For this review, take the finished solid that the model builds, in its own axes (mm). A direction names the side the tool comes from. Round coordinates to 2 decimals unless told otherwise and drop trailing zeros. Order: outer loops, then holes, each group sorted by start corner. A loop starts at its lowest first (then second) coordinate and runs counter-clockwise, first axis right, second up. Notation, with made-up numbers: (64.25, -6.5) -> (100.25, -6.5) arc R11 ccw to (100.25, 9.5) -> close; hole circle Ø6 at (70.25, 85). An arc over 180 degrees is marked (long way). Answer in a Markdown table with one row per item.
```python
from build123d import *

# Parameters (mm, degrees)
SKETCH1_W                = 18
SKETCH1_H                = 21
BOSS_EXTRUDE1_DEPTH      = 20
CUT_EXTRUDE3_DEPTH       = 30
CUT_EXTRUDE4_DEPTH       = 27
SKETCH6_W                = 20
SKETCH6_H                = 17
CUT_EXTRUDE5_DEPTH       = 17
SKETCH9_W                = 17
SKETCH9_H                = 4
CUT_EXTRUDE7_DEPTH       = 4
SKETCH10_W               = 20
SKETCH10_H               = 4
CUT_EXTRUDE8_DEPTH       = 30
BOSS_EXTRUDE3_DEPTH      = 4
SKETCH13_W               = 18
SKETCH13_H               = 1.5
SKETCH13_W_2             = 20
CUT_EXTRUDE11_DEPTH      = 21
CUT_EXTRUDE12_DEPTH      = 26
SKETCH16_R               = 1.9
BOSS_EXTRUDE4_DEPTH      = 14.5
SKETCH22_R               = 1.25
CUT_EXTRUDE15_DEPTH      = 19
CUT_EXTRUDE15_DEPTH_BACK = 27
CHAMFER1_SIZE            = 1.5
SKETCH23_W               = 18
SKETCH23_H               = 5
CUT_EXTRUDE16_DEPTH      = 4
SKETCH24_R               = 2
BOSS_EXTRUDE7_DEPTH      = 29
BOSS_EXTRUDE8_REACH      = 31
SKETCH25_W               = 4.5
SKETCH25_H               = 5.9
SKETCH26_R               = 1.6
CUT_EXTRUDE17_DEPTH      = 10


with BuildPart() as part:
    # Sketch1 → Boss-Extrude1 (new body)
    with BuildSketch(Plane(origin=(0, 0, 0), x_dir=(1, 0, 0), z_dir=(0, 1, 0))):
        Polygon((17.5, 14.5), (-8.5, 14.5), (-8.5, -14.5), (17.5, -14.5), (17.5, -10.5), (17.5, 10.5), align=None)
        with Locations((26.5, 0)):
            Rectangle(SKETCH1_W, SKETCH1_H)
    extrude(amount=BOSS_EXTRUDE1_DEPTH)

    # Sketch3 → Cut-Extrude3 (cut, through all)
    with BuildSketch(Plane.XY.offset(14.5)):
        Polygon((-8.5, 20), (-8.5, 18.5), (-4.5, 20), align=None)
    extrude(amount=-CUT_EXTRUDE3_DEPTH, mode=Mode.SUBTRACT)

    # Sketch4 → Cut-Extrude4 (cut, through all)
    with BuildSketch(Plane(origin=(17.5, 0, 0), x_dir=(0, 0, -1), z_dir=(1, 0, 0))):
        Polygon((-14.5, 20), (-14.5, 18.5), (-11.5, 20), align=None)
        Polygon((14.5, 20), (11.5, 20), (14.5, 18.5), align=None)
    extrude(amount=-CUT_EXTRUDE4_DEPTH, mode=Mode.SUBTRACT)

    # Sketch6 → Cut-Extrude5 (cut)
    with BuildSketch(Plane.XZ):
        with Locations((4.5, 0)):
            Rectangle(SKETCH6_W, SKETCH6_H)
    extrude(amount=-CUT_EXTRUDE5_DEPTH, mode=Mode.SUBTRACT)

    # Sketch9 → Cut-Extrude7 (cut)
    with BuildSketch(Plane.ZY.offset(8.5)):
        with Locations((0, 15)):
            Rectangle(SKETCH9_W, SKETCH9_H)
    extrude(amount=-CUT_EXTRUDE7_DEPTH, mode=Mode.SUBTRACT)

    # Sketch10 → Cut-Extrude8 (cut, through all)
    with BuildSketch(Plane.XY.offset(14.5)):
        with Locations((4.5, 12)):
            Rectangle(SKETCH10_W, SKETCH10_H)
    extrude(amount=-CUT_EXTRUDE8_DEPTH, mode=Mode.SUBTRACT)

    # Sketch12 → Boss-Extrude3 (add)
    with BuildSketch(Plane.XY.offset(14.5)):
        Polygon((22.5, 1.4), (34.5, 1.4), (34.5, 0), (34.5, -2), (29.5, -5), (12.5, -5), (7.5, 0), (17.5, 0), (17.5, 5), align=None)
    boss_extrude3 = extrude(amount=-BOSS_EXTRUDE3_DEPTH)

    # Mirror1: Boss-Extrude3 across plane
    add(boss_extrude3.mirror(Plane.XY))

    # Sketch13 → Cut-Extrude11 (cut)
    with BuildSketch(Plane.XY.offset(10.5)):
        with Locations((26.5, 19.25)):
            Rectangle(SKETCH13_W, SKETCH13_H)
        with Locations((25.5, 0.75)):
            Rectangle(SKETCH13_W_2, SKETCH13_H)
    extrude(amount=-CUT_EXTRUDE11_DEPTH, mode=Mode.SUBTRACT)

    # Sketch14 → Cut-Extrude12 (cut, through all)
    with BuildSketch(Plane.XY.offset(10.5)):
        with BuildLine():
            ThreePointArc((35.5, 10), (33.01040764, 3.98959236), (27, 1.5))
            Line((27, 1.5), (35.5, 1.5))
            Line((35.5, 1.5), (35.5, 10))
        make_face()
        with BuildLine():
            Line((35.5, 18.5), (27, 18.5))
            ThreePointArc((27, 18.5), (33.01040764, 16.01040764), (35.5, 10))
            Line((35.5, 10), (35.5, 18.5))
        make_face()
    extrude(amount=-CUT_EXTRUDE12_DEPTH, mode=Mode.SUBTRACT)

    # Sketch16 → Boss-Extrude4 (add, symmetric)
    with BuildSketch(Plane.XY):
        with Locations((27, 10)):
            Circle(SKETCH16_R)
    extrude(amount=BOSS_EXTRUDE4_DEPTH, both=True)

    # Sketch22 → Cut-Extrude15 (cut, two sides)
    with BuildSketch(Plane(origin=(17.5, 0, 0), x_dir=(0, 0, -1), z_dir=(1, 0, 0))) as cut_extrude15_sk:
        with Locations((0, 15.75)):
            Circle(SKETCH22_R)
    extrude(amount=CUT_EXTRUDE15_DEPTH, mode=Mode.SUBTRACT)
    extrude(cut_extrude15_sk.sketch, amount=-CUT_EXTRUDE15_DEPTH_BACK, mode=Mode.SUBTRACT)

    # Chamfer1
    chamfer1_edges = [part.edges().sort_by_distance(p)[0] for p in [
        (22.25, 18.5, -10.5),
        (22.25, 18.5, 10.5),
        (24.680555556, 1.5, 10.5),
        (24.680555556, 1.5, -10.5),
        (35.5, 10, -10.5),
        (35.5, 10, 10.5),
    ]]
    chamfer(chamfer1_edges, length=CHAMFER1_SIZE)

    # Sketch23 → Cut-Extrude16 (cut)
    with BuildSketch(Plane(origin=(0, 18.5, 0), x_dir=(1, 0, 0), z_dir=(0, 1, 0))):
        with Locations((26.5, 0)):
            Rectangle(SKETCH23_W, SKETCH23_H)
    extrude(amount=-CUT_EXTRUDE16_DEPTH, mode=Mode.SUBTRACT)

    # Sketch24 → Boss-Extrude7 (add, through all)
    with BuildSketch(Plane.XY.offset(14.5)):
        with Locations((3.5, 0)):
            Circle(SKETCH24_R)
    extrude(amount=-BOSS_EXTRUDE7_DEPTH)

    # Sketch25 → Boss-Extrude8 (add, up to next)
    with BuildSketch(Plane.XY.offset(14.5), mode=Mode.PRIVATE) as boss_extrude8_sk1:
        with Locations((27.25, -2.05)):
            Rectangle(SKETCH25_W, SKETCH25_H)
    boss_extrude8_tool1 = extrude(boss_extrude8_sk1.sketch, amount=-BOSS_EXTRUDE8_REACH, mode=Mode.PRIVATE) - part.part
    add(boss_extrude8_tool1.solids().sort_by_distance((27.25, -2.05, 14.5))[0])

    # Sketch26 → Cut-Extrude17 (cut)
    with BuildSketch(Plane(origin=(29.5, 0, 0), x_dir=(0, 0, -1), z_dir=(1, 0, 0))):
        with Locations((0, -2.05)):
            Circle(SKETCH26_R)
    extrude(amount=-CUT_EXTRUDE17_DEPTH, mode=Mode.SUBTRACT)


solid = part.part
```
Q1. Take a section at A-A, the plane x = 3.5. Write out the cut boundary in (y, z), then the cut area to 4 significant figures.
Answer key:
| item | result |
|---|---|
| outline | (-2, -14.5) -> (10, -14.5) -> (10, -8.5) -> (2, -8.5) -> (2, 8.5) -> (10, 8.5) -> (10, 14.5) -> (-2, 14.5) -> close; (14, -14.5) -> (18.5, -14.5) -> (20, -11.5) -> (20, 11.5) -> (18.5, 14.5) -> (14, 14.5) -> (14, 8.5) -> (17, 8.5) -> (17, -8.5) -> (14, -8.5) -> close |
| area | 330.5 mm^2 |
Q2. Tool access review of faces 1 (the face through (4, 10, -11)), 2 (the face through (21, 1.5, 0)), 3 (the face through (25, 0, 0)), 4 (the face through (26, 14.5, 0)), 5 (the face through (14.5, 8, 0)): name each direction out of +Z, -Z, +X, -X, +Y, -Y from which nothing blocks a thin tool from reaching the whole face with its end or side.
Answer key:
| item | result |
|---|---|
| face 1 | +Z, -Z |
| face 2 | +X |
| face 3 | -Y |
| face 4 | +X, +Y |
| face 5 | none |
Q3. Clearance check with flat-ended pins moving along their axes: pin 1 Ø13.5 at (x, z) = (1.5, 0) entering from -Y; pin 2 Ø3 at (x, y) = (26.5, 16) entering from +Z; pin 3 Ø1 at (y, z) = (0, 13) entering from +X. State where each tip first meets the part, or that it passes through.
Answer key:
| item | result |
|---|---|
| pin 1 | stops at y = -2 |
| pin 2 | stops at z = 10.5 |
| pin 3 | stops at x = 34.5 |
Q4. The part is to be moulded in two halves that separate along Y. For faces 6 (the face through (29.5, 0, 0)), 7 (the face through (22, 18.5, 6)), 8 (the face through (28, 1.4, 13)), say which applies: +Y half, -Y half, draft (parallel to the pull), parting line (faces both ways), or undercut.
Answer key:
| item | result |
|---|---|
| face 6 | draft |
| face 7 | +Y half |
| face 8 | undercut |
Q5. To check wall thickness, follow probe 1 along Y at (x, z) = (26.05, 0); probe 2 along Z at (x, y) = (13, 14.75); probe 3 along Z at (x, y) = (15.95, 15.75). State the ranges of each line that lie inside material, in increasing order.
Answer key:
| item | result |
|---|---|
| probe 1 | y = -5 to -3.65, -0.45 to 0.9, 1.5 to 14.5 |
| probe 2 | z = -14.5 to -8.5, 8.5 to 14.5 |
| probe 3 | z = -14.5 to -1.25, 1.25 to 14.5 |
Q6. Take a section at D-D, the plane x = 31. Give the number of separate pieces and of enclosed holes in the cut face, then the cut area to 3 significant figures.
Answer key:
| item | result |
|---|---|
| separate pieces | 3 |
| enclosed holes | 0 |
| area | 339 mm^2 |
Q7. Take a section at C-C, the plane x = 16. Write out the cut boundary in (y, z).
Answer key:
| item | result |
|---|---|
| outline | (-5, -14.5) -> (18.5, -14.5) -> (20, -11.5) -> (20, 11.5) -> (18.5, 14.5) -> (-5, 14.5) -> (-5, 10.5) -> (1.5, 10.5) -> (1.5, -10.5) -> (-5, -10.5) -> close; hole circle Ø2.5 at (15.75, 0) |
Q8. Take a section at B-B, the plane z = 7. Write out the cut boundary in (x, y), then the cut area to 3 significant figures.
Answer key:
| item | result |
|---|---|
| outline | (-8.5, 0) -> (-5.5, 0) -> (-5.5, 13) -> (-8.5, 13) -> close; (-8.5, 17) -> (14.5, 17) -> (14.5, 0) -> (15.5, 0) -> (15.5, 1.5) -> (27, 1.5) arc R8.5 ccw to (27, 18.5) -> (17.5, 18.5) -> (17.5, 20) -> (-4.5, 20) -> (-8.5, 18.5) -> close; circle Ø4 at (3.5, 0); (25, -5) -> (29.5, -5) -> (29.5, 0.9) -> (25, 0.9) -> close |
| area | 476 mm^2 |
